Geometry check sheet. Reference: the model listing, model coordinates, mm. Face numbers are marked on the shaded views. Coordinates: 2 decimals unless noted, no trailing zeros. Order: outer loops, then holes, each group sorted by start corner. A loop starts at its lowest first (then second) coordinate and runs counter-clockwise, first axis right, second up. Notation, with made-up numbers: (8.25, 18.25) - (67.25, 18.25) arc R9 cw to (67.25, 27.25) - close; hole circle Ø10 at (80, -3.5). An arc over 180 degrees is marked (long way). Return JSON: item names as keys, results as strings. Group by question number.
Item 1: Draft check along Y on the marked faces 1 and 2. Enter one of: pulls with the +Y half, pulls with the -Y half, needs draft (parallel to the pull), parting line crosses it, or undercut.
Item 2: Section check A-A on z = 3.15. Enter the section's corners in (x, y).
Item 3: Gauge pin test, flat end, axial feed: pin 1 (1.5 mm diameter, centred on y = -6.5, z = 1, fed in from +X). Record the tip position at first contact, or that the pin passes through.
Item 4: Scan lines: probe 1 along Y at (x, z) = (3.25, 1.5); probe 2 along X at (y, z) = (1, 0.65); probe 3 along Y at (x, z) = (0, 1.5). Record each from-to range of solid material in increasing order.
from build123d import *

# Parameters (mm, degrees)
SKETCH1_R             = 11.5
SKETCH1_R_2           = 10.5
BOSS_EXTRUDE1_DEPTH   = 4
SKETCH1_R_3           = 9.5
SKETCH1_R_4           = 8.5
BOSS_EXTRUDE1_2_DEPTH = 4
CHAMFER1_SIZE         = 0.2
CHAMFER2_SIZE         = 0.2
SKETCH1_3_R           = 10.5
SKETCH1_3_R_2         = 9.5
BOSS_EXTRUDE2_DEPTH   = 4


with BuildPart() as part:
    # Sketch1 → Boss-Extrude1 (new body)
    with BuildSketch(Plane.XY):
        Circle(SKETCH1_R)
        Circle(SKETCH1_R_2, mode=Mode.SUBTRACT)
    extrude(amount=BOSS_EXTRUDE1_DEPTH)

    # Chamfer1
    chamfer1_edges = [part.edges().sort_by_distance(p)[0] for p in [
        (-11.5, 0, 0),
        (-10.5, 0, 0),
        (-10.5, 0, 4),
        (-11.5, 0, 4),
    ]]
    chamfer(chamfer1_edges, length=CHAMFER1_SIZE)



with BuildPart() as body_2:
    # Sketch1 → Boss-Extrude1 2 (new body)
    with BuildSketch(Plane.XY):
        Circle(SKETCH1_R_3)
        Circle(SKETCH1_R_4, mode=Mode.SUBTRACT)
    extrude(amount=BOSS_EXTRUDE1_2_DEPTH)

    # Chamfer2
    chamfer2_edges = [body_2.edges().sort_by_distance(p)[0] for p in [
        (-9.5, 0, 0),
        (-8.5, 0, 0),
        (-8.5, 0, 4),
        (-9.5, 0, 4),
    ]]
    chamfer(chamfer2_edges, length=CHAMFER2_SIZE)


with BuildPart() as part_1:
    add(part.part)

    add(body_2.part)  # Boss-Extrude2 merges body 2
    # Sketch1<3> → Boss-Extrude2 (add)
    with BuildSketch(Plane.XY):
        Circle(SKETCH1_3_R)
        Circle(SKETCH1_3_R_2, mode=Mode.SUBTRACT)
    extrude(amount=BOSS_EXTRUDE2_DEPTH)


solid = part_1.part
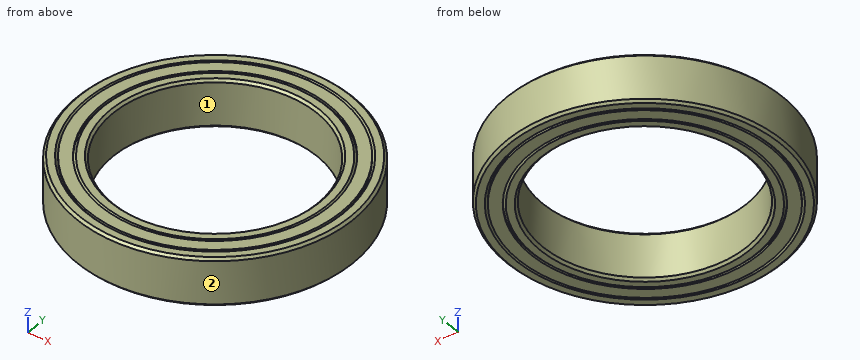
Computed:
{
 "1": {"face 1": "undercut", "face 2": "parting line crosses it"},
 "2": {"outline": "circle Ø23 at (0, 0); hole circle Ø17 at (0, 0)"},
 "3": {"pin 1": "stops at x = 9.96"},
 "4": {"probe 1": "y = -11.03 to -7.85, 7.85 to 11.03", "probe 2": "x = -11.46 to -8.44, 8.44 to 11.46", "probe 3": "y = -11.5 to -8.5, 8.5 to 11.5"}
}
